```python
from build123d import *

# Parameters (mm, degrees)
SKETCH1_W           = 55
SKETCH1_H           = 65
BOSS_EXTRUDE1_DEPTH = 13
SKETCH2_W           = 30
SKETCH2_H           = 45
BOSS_EXTRUDE2_DEPTH = 50
SKETCH5_R           = 20.5
CUT_EXTRUDE1_DEPTH  = 26
SKETCH7_R           = 7
CUT_EXTRUDE2_DEPTH  = 20
SKETCH8_R           = 2.25
CUT_EXTRUDE3_DEPTH  = 20
FILLET2_R           = 10
SKETCH9_W           = 30
SKETCH9_H           = 45
CUT_EXTRUDE4_DEPTH  = 5
FILLET3_R           = 10
FILLET4_R           = 10


with BuildPart() as part:
    # Sketch1 → Boss-Extrude1 (new body)
    with BuildSketch(Plane(origin=(0, 0, 0), x_dir=(1, 0, 0), z_dir=(0, 1, 0))):
        with Locations((-5, 0)):
            Rectangle(SKETCH1_W, SKETCH1_H)
    extrude(amount=BOSS_EXTRUDE1_DEPTH)

    # Sketch2 → Boss-Extrude2 (add)
    with BuildSketch(Plane(origin=(0, 13, 0), x_dir=(1, 0, 0), z_dir=(0, 1, 0))):
        with Locations((7.5, 0)):
            Rectangle(SKETCH2_W, SKETCH2_H)
    extrude(amount=BOSS_EXTRUDE2_DEPTH)

    # Sketch5 → Cut-Extrude1 (cut)
    with BuildSketch(Plane(origin=(22.5, 0, 0), x_dir=(0, 0, -1), z_dir=(1, 0, 0))):
        with Locations((0, 35)):
            Circle(SKETCH5_R)
    extrude(amount=-CUT_EXTRUDE1_DEPTH, mode=Mode.SUBTRACT)

    # Sketch7 → Cut-Extrude2 (cut)
    with BuildSketch(Plane(origin=(-3.5, 0, 0), x_dir=(0, 0, -1), z_dir=(1, 0, 0))):
        with Locations((0, 35)):
            Circle(SKETCH7_R)
    extrude(amount=-CUT_EXTRUDE2_DEPTH, mode=Mode.SUBTRACT)

    # Sketch8 → Cut-Extrude3 (cut)
    with BuildSketch(Plane(origin=(0, 0, 0), x_dir=(-1, 0, 0), z_dir=(0, -1, 0))):
        with Locations(Location((12.5, -22.5, 0), (0, 0, 90))):
            Circle(SKETCH8_R)
        with Locations(Location((12.5, 22.5, 0), (0, 0, 90))):
            Circle(SKETCH8_R)
        with Locations(Location((-12.5, 22.5, 0), (0, 0, 90))):
            Circle(SKETCH8_R)
        with Locations(Location((-12.5, -22.5, 0), (0, 0, 90))):
            Circle(SKETCH8_R)
    extrude(amount=-CUT_EXTRUDE3_DEPTH, mode=Mode.SUBTRACT)

    # Fillet2
    fillet2_edges = [part.edges().sort_by_distance(p)[0] for p in [
        (-32.5, 6.5, 32.5),
    ]]
    fillet(fillet2_edges, radius=FILLET2_R)

    # Sketch9 → Cut-Extrude4 (cut)
    with BuildSketch(Plane(origin=(0, 63, 0), x_dir=(1, 0, 0), z_dir=(0, 1, 0))):
        with Locations((7.5, 0)):
            Rectangle(SKETCH9_W, SKETCH9_H)
    extrude(amount=-CUT_EXTRUDE4_DEPTH, mode=Mode.SUBTRACT)

    # Fillet3
    fillet3_edges = [part.edges().sort_by_distance(p)[0] for p in [
        (7.5, 58, 22.5),
    ]]
    fillet(fillet3_edges, radius=FILLET3_R)

    # Fillet4
    fillet4_edges = [part.edges().sort_by_distance(p)[0] for p in [
        (7.5, 58, -22.5),
    ]]
    fillet(fillet4_edges, radius=FILLET4_R)


solid = part.part
```
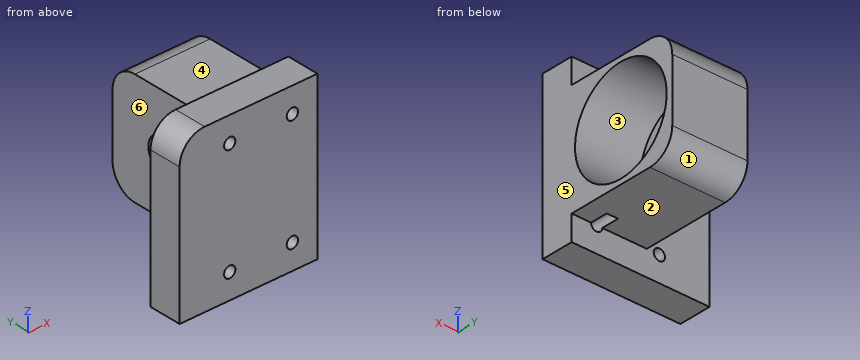
Input: part model. Units: mm. Frame: model coordinates. Face numbers are marked on the shaded views. A direction names the side the tool comes from. Give positions to 0.01 mm unless a question says otherwise; leave off trailing zeros. Order: outer loops, then holes, each group sorted by start corner. A loop starts at its lowest first (then second) coordinate and runs counter-clockwise, first axis right, second up. Notation, with made-up numbers: (42, 88.25) -> (49, 88.25) arc R3 cw to (49, 93.25) -> close; hole circle Ø8 at (83.5, -17). An arc over 180 degrees is marked (long way). Write each question's results on one line, items separated by ' | '. Start each with the question number.
Item 1: Cut plane B-B on x = 12.5. Return the cut outline in (y, z), then the cut area to 3 significant figures.
Item 2: Cut plane C-C on x = -12.5. Return the cut outline in (y, z), then the cut area to 3 significant figures.
Item 3: Contact query for flat-ended pins moving along their axis: P1, Ø9, axis at x = 11, y = 24, coming from the +Z side; P2, Ø6, axis at x = -12.5, z = 22.5, coming from the +Y side; P3, Ø22.5, axis at y = 35, z = 0, coming from the +X side. Output: stop coordinate, or through.
Item 4: Cut plane A-A on z = 0. Return the cut outline in (x, y), then the cut area to 3 significant figures.
Item 5: Mould query, pull axis Y, two halves, no side actions, for the marked faces 1, 2 and 3. Classes: pulls with the +Y half, pulls with the -Y half, needs draft (parallel to the pull), parting line crosses it, or undercut.
Item 6: Set-up query: the marked faces 4, 5 and 6. Return all of +Z, -Z, +X, -X, +Y, -Y with unobstructed straight access to the full face (end or side cutting, diameter ignored); none if empty.
Item 7: Cut plane D-D on y = 35. Return the cut outline in (x, z), then the cut area to 3 significant figures.
Item 8: Line query: line 1 (X direction, y = 8.5, z = 22.5); line 2 (Z direction, x = 12.5, y = 12.5); line 3 (Z direction, x = -0.5, y = 35.5). Output: solid intervals per line, ascending.
Established:
1) outline: (0, -32.5) -> (13, -32.5) -> (13, -24.75) -> (0, -24.75) -> close; (0, -20.25) -> (20, -20.25) -> (20, -22.5) -> (48, -22.5) arc R10 ccw to (58, -12.5) -> (58, 12.5) arc R10 ccw to (48, 22.5) -> (20, 22.5) -> (20, 20.25) -> (0, 20.25) -> close; (0, 24.75) -> (13, 24.75) -> (13, 32.5) -> (0, 32.5) -> close; hole circle Ø41 at (35, 0) | area: 1,360 mm^2
2) outline: (0, -32.5) -> (13, -32.5) -> (13, -24.75) -> (0, -24.75) -> close; (0, -20.25) -> (13, -20.25) -> (13, 20.25) -> (0, 20.25) -> close; (0, 24.75) -> (13, 24.75) -> (13, 32.5) -> (0, 32.5) -> close | area: 728 mm^2
3) P1: z = 22.5 | P2: y = 13 | P3: x = -3.5
4) outline: (-32.5, 0) -> (22.5, 0) -> (22.5, 14.5) -> (-3.5, 14.5) -> (-3.5, 28) -> (-7.5, 28) -> (-7.5, 13) -> (-32.5, 13) -> close; (-7.5, 42) -> (-3.5, 42) -> (-3.5, 55.5) -> (22.5, 55.5) -> (22.5, 58) -> (-7.5, 58) -> close | area: 943 mm^2
5) face 1: pulls with the +Y half | face 2: needs draft | face 3: undercut
6) face 4: +Z, +X, -X, +Y | face 5: +Z, -Z, +X, +Y, -Y | face 6: +Z, -Z, -X, +Y
7) outline: (-7.5, -22.5) -> (22.5, -22.5) -> (22.5, -20.5) -> (-3.5, -20.5) -> (-3.5, -7) -> (-7.5, -7) -> close; (-7.5, 7) -> (-3.5, 7) -> (-3.5, 20.5) -> (22.5, 20.5) -> (22.5, 22.5) -> (-7.5, 22.5) -> close | area: 228 mm^2
8) line 1: -32.5 to -14.75, -10.25 to 10.25, 14.75 to 22.5 | line 2: -32.5 to -24.75, -20.25 to 20.25, 24.75 to 32.5 | line 3: -22.5 to -20.49, 20.49 to 22.5
